CAD build for the part. Positions are in the model's coordinates, mm. Coordinates: 2 decimals unless noted, no trailing zeros.
```python
from build123d import *

# Parameters (mm, degrees)
SKETCH1_R           = 15
SKETCH1_W           = 9.033789511
SKETCH1_H           = 25.11797261
BOSS_EXTRUDE1_DEPTH = 3


with BuildPart() as part:
    # Sketch1 → Boss-Extrude1 (new body)
    with BuildSketch(Plane(origin=(0, 0, 0), x_dir=(1, 0, 0), z_dir=(0, 1, 0))):
        with BuildLine():
            add(Edge.make_bspline(
                [(-25.850267552, 0), (-0.763553632, -79.235152429), (24.323160288, 0)],
                knots=[0, 0, 0, 1, 1, 1], degree=2))
            add(Edge.make_bspline(
                [(24.323160288, 0), (67.143381198, 26.049823561), (68.440320284, 60.482028786), (-0.763553632, 60)],
                knots=[0, 0, 0, 0, 1, 1, 1, 1], degree=3))
            add(Edge.make_bspline(
                [(-25.850267552, 0), (-68.670488462, 26.049823561), (-69.967427548, 60.482028786), (-0.763553632, 60)],
                knots=[0, 0, 0, 0, 1, 1, 1, 1], degree=3))
        make_face()
        with Locations(Location((-0.763553632, -15.237324398, 0), (0, 0, 270))):
            Circle(SKETCH1_R, mode=Mode.SUBTRACT)
        with Locations((39.236446368, 35)):
            Rectangle(SKETCH1_W, SKETCH1_H, mode=Mode.SUBTRACT)
        with Locations((-40.763553633, 35)):
            Rectangle(SKETCH1_W, SKETCH1_H, mode=Mode.SUBTRACT)
    extrude(amount=BOSS_EXTRUDE1_DEPTH)


solid = part.part
```
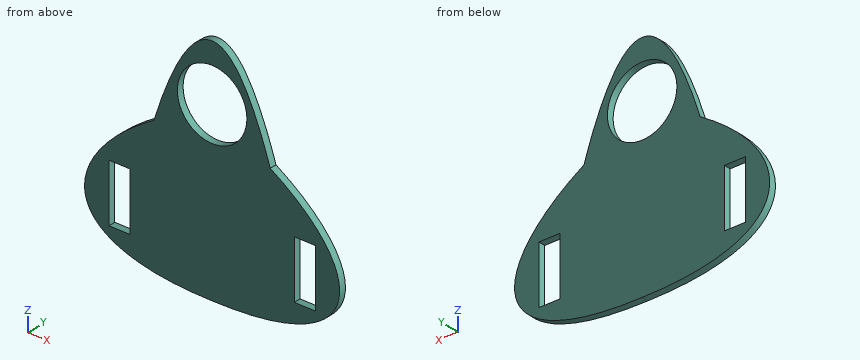
Item 1: Flat gauge pins, fed straight in: pin 1 Ø1.5 at (y, z) = (2, 3) entering from +X; pin 2 Ø0.9 at (y, z) = (1, -30.5) entering from -X; pin 3 Ø0.9 at (x, y) = (-43, 2) entering from +Z. Where does each tip first touch, or does it go through?
Item 2: Saw through at A-A, the plane y = 1.95. State how many separate pieces and enclosed holes the cut face has, and give its area (3 significant figures).
Item 3: Wall check: line 1 along X through (y, z) = (2.8, -26.5); line 2 along X through (y, z) = (0.5, -47); line 3 along Z through (x, y) = (-42, 2.3). Give the ranges that are in metal, low to high.
Working result:
1. pin 1: stops at x = 23.6
1. pin 2: stops at x = -55.09
1. pin 3: stops at z = -12.45
2. separate pieces: 1
2. enclosed holes: 3
2. area: 5,570 mm2
3. line 1: x = -53.41 to -45.28, -36.25 to 34.72, 43.75 to 51.89
3. line 2: x = -51.46 to -45.28, -36.25 to 34.72, 43.75 to 49.94
3. line 3: z = -53.59 to -47.56, -22.44 to -11.94
